from build123d import *

# Parameters (mm, degrees)
EXTRUDE_1_DEPTH          = 10
FILLET_1_R               = 2
SKETCH_2_R               = 1.55
CUT_EXTRUDE_1_DEPTH      = 11
SKETCH_3_W               = 30
SKETCH_3_H               = 5
CUT_EXTRUDE_2_DEPTH      = 1
CUT_EXTRUDE_2_DEPTH_BACK = 11
FILLET_2_R               = 3
SKETCH_5_R               = 3.5
CUT_EXTRUDE_3_DEPTH      = 4


with BuildPart() as part:
    # 草图1 → 凸台-拉伸1 (new body)
    with BuildSketch(Plane.XY):
        Polygon((7.25, 0), (-7.25, 0), (-7.25, 5), (-15, 5), (-15, -15), (15, -15), (15, 5), (7.25, 5), align=None)
    extrude(amount=EXTRUDE_1_DEPTH)

    # 圆角1
    fillet_1_edges = [part.edges().sort_by_distance(p)[0] for p in [
        (15, 5, 5),
        (15, -15, 5),
        (-15, -15, 5),
        (-15, 5, 5),
    ]]
    fillet(fillet_1_edges, radius=FILLET_1_R)

    # 草图2 → 切除-拉伸1 (cut, through all)
    with BuildSketch(Plane.XY.offset(10)):
        with Locations((-6.5, -7.5)):
            Circle(SKETCH_2_R)
        with Locations((6.5, -7.5)):
            Circle(SKETCH_2_R)
    extrude(amount=-CUT_EXTRUDE_1_DEPTH, mode=Mode.SUBTRACT)

    # 草图3 → 切除-拉伸2 (cut, two sides)
    with BuildSketch(Plane.XY.offset(10)) as cut_extrude_2_sk:
        with Locations((0, 2.5)):
            Rectangle(SKETCH_3_W, SKETCH_3_H)
    extrude(amount=CUT_EXTRUDE_2_DEPTH, mode=Mode.SUBTRACT)
    extrude(cut_extrude_2_sk.sketch, amount=-CUT_EXTRUDE_2_DEPTH_BACK, mode=Mode.SUBTRACT)

    # 圆角2
    fillet_2_edges = [part.edges().sort_by_distance(p)[0] for p in [
        (15, 0, 5),
        (-15, 0, 5),
    ]]
    fillet(fillet_2_edges, radius=FILLET_2_R)

    # 草图5 → 切除-拉伸3 (cut)
    with BuildSketch(Plane.XY.offset(10)):
        with Locations((-6.5, -7.500000001)):
            Circle(SKETCH_5_R)
        with Locations((6.5, -7.5)):
            Circle(SKETCH_5_R)
    extrude(amount=-CUT_EXTRUDE_3_DEPTH, mode=Mode.SUBTRACT)


solid = part.part
Could you check a few things on this model? Use its own coordinates, in mm. A direction names the side the tool comes from. Coordinates: 2 decimals unless noted, no trailing zeros. Order: outer loops, then holes, each group sorted by start corner. A loop starts at its lowest first (then second) coordinate and runs counter-clockwise, first axis right, second up. Notation, with made-up numbers: (4.25, 65) - (21.25, 65) arc R31 ccw to (21.25, 100) - close; hole circle Ø1 at (-40, 64.25). An arc over 180 degrees is marked (long way). Answer in a Markdown table with one row per item. Add a question column.
(1) I need wall thicknesses on L1, parallel to Y at x = 6.5, z = 7.3; L2, parallel to Y at x = -6.5, z = 1.9; L3, parallel to X at y = -7.25, z = 6.5. Which ranges of each line are inside material? Lowest first, please.
(2) If we section it at C-C, the plane x = 6.75: Please give me the cut outline in (y, z), then the cut area to 3 significant figures.
(3) If we section it at B-B, the plane z = 2.5: Please give me the cut outline in (x, y), then the cut area to 3 significant figures.
(4) On a 3-axis mill with a long thin cutter (end or side, diameter ignored), from which of +Z, -Z, +X, -X, +Y, -Y can I reach the whole of each face in a straight line? I mean faces 1 (the face through (-4.99, -6.67, 6)), 2 (the face through (0, -7, 10)). Say none if no direction works.
(5) If we section it at D-D, the plane x = -6.5: Please give me the cut outline in (y, z).
(6) If we section it at A-A, the plane y = -7.5: Please give me the cut outline in (x, z).
(7) If we mould it in two halves opening along Y, with no side actions, what happens to faces 3 (the face through (5.27, -8.44, 3.04)), 4 (the face through (-6.836, -9.013, 3.042)), 5 (the face through (-15, -8, 5)), 6 (the face through (0, 0, 5))? For each: released by +Y, released by -Y, zero draft, split by the parting line, or undercut.
(8) Will this pin go through, and if not, where does the flat tip stop? pin 1 (4 mm diameter, centred on x = -6.5, y = -7.5, fed in from +Z).
Results are:
| question | item | result |
|---|---|---|
| 1 | L1 | y = -15 to -11, -4 to 0 |
| 1 | L2 | y = -15 to -9.05, -5.95 to 0 |
| 1 | L3 | x = -15 to -9.99, -3.01 to 3.01, 9.99 to 15 |
| 2 | outline | (-15, 0) - (-9.03, 0) - (-9.03, 6) - (-10.99, 6) - (-10.99, 10) - (-15, 10) - close; (-5.97, 0) - (0, 0) - (0, 10) - (-4.01, 10) - (-4.01, 6) - (-5.97, 6) - close |
| 2 | area | 104 mm2 |
| 3 | outline | (-15, -13) arc R2 ccw to (-13, -15) - (13, -15) arc R2 ccw to (15, -13) - (15, -3) arc R3 ccw to (12, 0) - (-12, 0) arc R3 ccw to (-15, -3) - close; hole circle Ø3.1 at (-6.5, -7.5); hole circle Ø3.1 at (6.5, -7.5) |
| 3 | area | 429 mm2 |
| 4 | face 1 | +Z |
| 4 | face 2 | +Z, +X, -X, +Y, -Y |
| 5 | outline | (-15, 0) - (-9.05, 0) - (-9.05, 6) - (-11, 6) - (-11, 10) - (-15, 10) - close; (-5.95, 0) - (0, 0) - (0, 10) - (-4, 10) - (-4, 6) - (-5.95, 6) - close |
| 6 | outline | (-15, 0) - (-8.05, 0) - (-8.05, 6) - (-10, 6) - (-10, 10) - (-15, 10) - close; (-4.95, 0) - (4.95, 0) - (4.95, 6) - (3, 6) - (3, 10) - (-3, 10) - (-3, 6) - (-4.95, 6) - close; (8.05, 0) - (15, 0) - (15, 10) - (10, 10) - (10, 6) - (8.05, 6) - close |
| 7 | face 3 | undercut |
| 7 | face 4 | undercut |
| 7 | face 5 | zero draft |
| 7 | face 6 | released by +Y |
| 8 | pin 1 | stops at z = 6 |
